from build123d import *

# Parameters (mm, degrees)
SKETCH1_R                = 12.0269
BOSS_EXTRUDE1_DEPTH      = 65.8876
BOSS_EXTRUDE2_DEPTH      = 23.0124
BOSS_EXTRUDE2_DEPTH_BACK = 88.9
SKETCH2_W                = 3.175
SKETCH2_H                = 19.05
CUT_EXTRUDE1_DEPTH       = 23.0124
CUT_EXTRUDE2_DEPTH       = 23.0124


with BuildPart() as part:
    # Sketch1 → Boss-Extrude1 (new body)
    with BuildSketch(Plane(origin=(0, 0, 0), x_dir=(0, 0, -1), z_dir=(1, 0, 0))):
        Circle(SKETCH1_R)
    extrude(amount=BOSS_EXTRUDE1_DEPTH)

    # Sketch2 → Boss-Extrude2 (add, two sides: drawn at the far end of the back side and taken through both)
    with BuildSketch(Plane(origin=(65.8876, 0, 0), x_dir=(0, 0, -1), z_dir=(1, 0, 0)).offset(-BOSS_EXTRUDE2_DEPTH_BACK)):
        Rectangle(SKETCH2_W, SKETCH2_H)
    extrude(amount=BOSS_EXTRUDE2_DEPTH + BOSS_EXTRUDE2_DEPTH_BACK)

    # Sketch5 → Cut-Extrude1 (cut)
    with BuildSketch(Plane(origin=(0, 0, -1.5875), x_dir=(-1, 0, 0), z_dir=(0, 0, -1))):
        with BuildLine():
            Line((-78.9813, 4.3688), (-78.1939, 4.3688))
            ThreePointArc((-78.1939, 4.3688), (-73.8251, 0), (-78.1939, -4.3688))
            Line((-78.1939, -4.3688), (-78.9813, -4.3688))
            ThreePointArc((-78.9813, -4.3688), (-83.3501, 0), (-78.9813, 4.3688))
        make_face()
    extrude(amount=-CUT_EXTRUDE1_DEPTH, mode=Mode.SUBTRACT)

    # Sketch6 → Cut-Extrude2 (cut)
    with BuildSketch(Plane(origin=(0, 0, -1.5875), x_dir=(-1, 0, 0), z_dir=(0, 0, -1))):
        with BuildLine():
            Line((13.095, -4.37), (12.305, -4.37))
            ThreePointArc((12.305, -4.37), (7.935, 0), (12.305, 4.37))
            Line((12.305, 4.37), (13.095, 4.37))
            ThreePointArc((13.095, 4.37), (17.465, 0), (13.095, -4.37))
        make_face()
    extrude(amount=-CUT_EXTRUDE2_DEPTH, mode=Mode.SUBTRACT)


solid = part.part
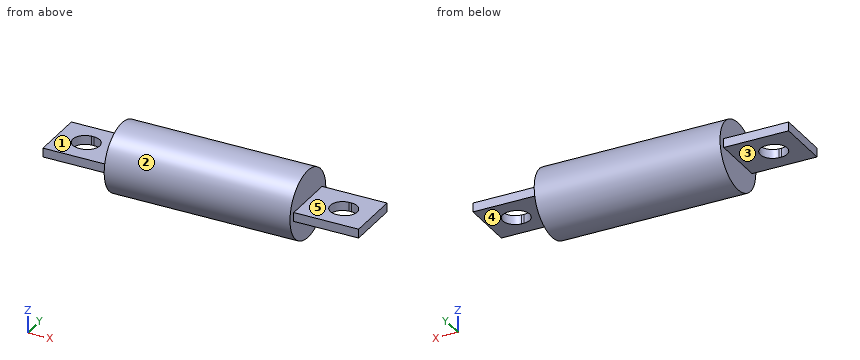
Source: CAD feature listing. Evaluate the final solid. Frame: model axes, mm. Face numbers are marked on the shaded views. A direction names the side the tool comes from. Give positions to 0.01 mm unless a question says otherwise; leave off trailing zeros. Write each loop counter-clockwise with the first axis right and the second up, starting at its lowest first coordinate (ties: lowest second). Pieces come first, ordered by that corner, then holes. Notation, with made-up numbers: (13.5, -31) -> (63.5, -31) arc R17 ccw to (63.5, -18) -> close; hole circle Ø7 at (-9.5, 6.5). An arc over 180 degrees is marked (long way). Write item = value, one per line.
Q1. Line query: line 1 (X direction, y = -10.75, z = 2.5); line 2 (Z direction, x = 4, y = 0.5); line 3 (Z direction, x = 73.5, y = -9). Output: solid intervals per line, ascending. Write a range as from..to.
Here are the results:
line_1 = 0..65.89
line_2 = -12.02..12.02
line_3 = -1.59..1.59
Q2. First-contact query: pin 1 (12 mm diameter, centred on x = 72, y = 0, fed in from +Z); pin 2 (6 mm diameter, centred on x = 74, y = 2.5, fed in from -Z); pin 3 (1.5 mm diameter, centred on x = 39, y = 1, fed in from +Z); pin 4 (7 mm diameter, centred on y = -4, z = 3, fed in from -X). Flat tips, straight axial feed; report the tip coordinate or a pass-through.
Here are the results:
pin_1 = 1.59
pin_2 = -1.59
pin_3 = 12.02
pin_4 = -23.01
Q3. Cut plane A-A on y = 0. Return loops of the section in (x, z) (1 decimal), then the cut area to 3 significant figures.
Here are the results:
outline = (-23, -1.6) -> (-17.5, -1.6) -> (-17.5, 1.6) -> (-23, 1.6) -> close; (-7.9, -1.6) -> (0, -1.6) -> (0, -12) -> (65.9, -12) -> (65.9, -1.6) -> (73.8, -1.6) -> (73.8, 1.6) -> (65.9, 1.6) -> (65.9, 12) -> (0, 12) -> (0, 1.6) -> (-7.9, 1.6) -> close; (83.4, -1.6) -> (88.9, -1.6) -> (88.9, 1.6) -> (83.4, 1.6) -> close
area = 1,670 mm²
Q4. Cut plane D-D on y = -7. Return loops of the section in (x, z).
Here are the results:
outline = (-23.01, -1.59) -> (0, -1.59) -> (0, -9.78) -> (65.89, -9.78) -> (65.89, -1.59) -> (88.9, -1.59) -> (88.9, 1.59) -> (65.89, 1.59) -> (65.89, 9.78) -> (0, 9.78) -> (0, 1.59) -> (-23.01, 1.59) -> close
Q5. Reachability of the marked faces 1, 2, 3, 4 and 5 from +Z, -Z, +X, -X, +Y, -Y: full face, straight path, thin tool, end or side. Return the list, or none.
Here are the results:
face_1 = +Z, -X, +Y, -Y
face_2 = +X, -X
face_3 = -Z, -X, +Y, -Y
face_4 = -Z, +X, +Y, -Y
face_5 = +Z, +X, +Y, -Y
Q6. Cut plane C-C on x = 19.5. Return loops of the section in (y, z), then the cut area to 3 significant figures.
Here are the results:
outline = circle Ø24.05 at (0, 0)
area = 454 mm²
Q7. Cut plane B-B on z = 0. Return loops of the section in (x, y) (3 decimals), then the cut area to 3 significant figures.
Here are the results:
outline = (-23.012, -9.525) -> (0, -9.525) -> (0, -12.027) -> (65.888, -12.027) -> (65.888, -9.525) -> (88.9, -9.525) -> (88.9, 9.525) -> (65.888, 9.525) -> (65.888, 12.027) -> (0, 12.027) -> (0, 9.525) -> (-23.012, 9.525) -> close; hole (-13.095, -4.37) -> (-12.305, -4.37) arc R4.37 ccw to (-12.305, 4.37) -> (-13.095, 4.37) arc R4.37 ccw to start; hole (78.194, -4.369) -> (78.981, -4.369) arc R4.369 ccw to (78.981, 4.369) -> (78.194, 4.369) arc R4.369 ccw to start
area = 2,330 mm²
